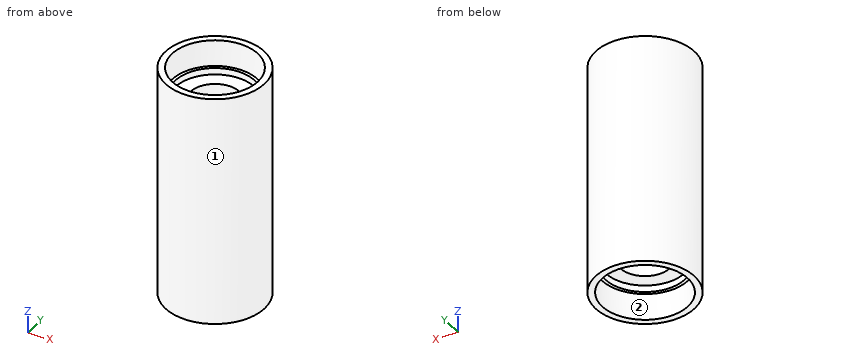
from build123d import *


with BuildPart() as part:
    # Эскиз1 → Повернуть1 (revolve)
    with BuildSketch(Plane(origin=(0, 0, 0), x_dir=(1, 0, 0), z_dir=(0, 1, 0))):
        Polygon((15, 0), (7.5, 0), (7.5, -24.990014613), (12, -24.990014613), (12, -26.990014613), (13, -26.990014613), (13, -34.990014613), (15, -34.990014613), align=None)
    revolve(axis=Axis((0, 0, 1005.29300139), (0, 0, -1)))

    # Зеркальное отражение1: part across plane


with BuildPart() as part_1:
    add(part.part)
    add(part.part.mirror(Plane(origin=(15, 0, 0), x_dir=(1, 0, 0), z_dir=(0, 0, -1))))


solid = part_1.part
Source: CAD feature listing. Evaluate the final solid. Frame: model axes, mm. Face numbers are marked on the shaded views. Coordinates: 2 decimals unless noted, no trailing zeros. Loops run counter-clockwise (first coordinate to the right, second up) from the corner with the lowest first, then second, coordinate; pieces in that order, holes last. Notation, with made-up numbers: (44, 37.25) - (82, 37.25) arc R16 ccw to (82, 46.25) - close; hole circle Ø7 at (38.25, 83). An arc over 180 degrees is marked (long way). Return JSON: item names as keys, results as strings.
Q1. Section A-A, the plane x = 0. Return loops of the section in (y, z), plus the area to 3 significant figures.
Results:
{"outline": "(-15, -34.99) - (-13, -34.99) - (-13, -26.99) - (-12, -26.99) - (-12, -24.99) - (-7.5, -24.99) - (-7.5, 24.99) - (-12, 24.99) - (-12, 26.99) - (-13, 26.99) - (-13, 34.99) - (-15, 34.99) - close; (7.5, -24.99) - (12, -24.99) - (12, -26.99) - (13, -26.99) - (13, -34.99) - (15, -34.99) - (15, 34.99) - (13, 34.99) - (13, 26.99) - (12, 26.99) - (12, 24.99) - (7.5, 24.99) - close", "area": "838 mm2"}
Q2. Material intervals for line 1 along Y through (x, z) = (0, 29.25); line 2 along Y through (x, z) = (0, -25.85), sorted ascending.
Results:
{"line 1": "-15 to -13, 13 to 15", "line 2": "-15 to -12, 12 to 15"}
Q3. Section C-C, the plane z = 23. Return loops of the section in (x, y).
Results:
{"outline": "circle Ø30 at (0, 0); hole circle Ø15 at (0, 0)"}
Q4. Section D-D, the plane y = -8.5. Return loops of the section in (x, z).
Results:
{"outline": "(-12.36, -34.99) - (-9.84, -34.99) - (-9.84, -26.99) - (-8.47, -26.99) - (-8.47, -24.99) - (8.47, -24.99) - (8.47, -26.99) - (9.84, -26.99) - (9.84, -34.99) - (12.36, -34.99) - (12.36, 34.99) - (9.84, 34.99) - (9.84, 26.99) - (8.47, 26.99) - (8.47, 24.99) - (-8.47, 24.99) - (-8.47, 26.99) - (-9.84, 26.99) - (-9.84, 34.99) - (-12.36, 34.99) - close"}
Q5. Contact query for flat-ended pins moving along their axis: P1, Ø1, axis at y = -4.5, z = -24, coming from the +X side; P2, Ø3, axis at y = 4, z = 26.5, coming from the -X side; P3, Ø14.5, axis at x = 0, y = 0, coming from the -Z side; P4, Ø17, axis at x = 0, y = 0, coming from the -Z side. Output: stop coordinate, or through.
Results:
{"P1": "x = 14.46", "P2": "x = -14.79", "P3": "through", "P4": "z = -24.99"}
Q6. Mould query, pull axis Y, two halves, no side actions, for the marked faces 1 and 2. Classes: released by +Y, released by -Y, zero draft, split by the parting line, or undercut.
Results:
{"face 1": "split by the parting line", "face 2": "undercut"}
